from build123d import *

# Parameters (mm, degrees)
F0_W           = 200
F0_H           = 200
F1_DEPTH       = 20
F2_R           = 2.5
F3_W           = 180
F3_H           = 180
F4_DEPTH       = 2
F6_D           = 8
F6_CBORE_D     = 13
F6_CBORE_DEPTH = 8


with BuildPart() as f1:
    # F0 (on Top) → F1 (new body)
    with BuildSketch(Plane.XY):
        Rectangle(F0_W, F0_H)
    extrude(amount=F1_DEPTH)

    # F2
    f2_edges = [f1.edges().sort_by_distance(p)[0] for p in [
        (0, 100, 20),
        (100, 0, 20),
        (100, 100, 10),
        (0, 100, 0),
        (100, 0, 0),
        (-100, 0, 0),
        (-100, 0, 20),
        (-100, 100, 10),
        (100, -100, 10),
        (0, -100, 20),
        (0, -100, 0),
        (-100, -100, 10),
    ]]
    fillet(f2_edges, radius=F2_R)

    # F3 (on face) → F4 (cut)
    with BuildSketch(Plane.XY.offset(20)):
        Rectangle(F3_W, F3_H)
    extrude(amount=-F4_DEPTH, mode=Mode.SUBTRACT)

    # F6 (through all)
    with Locations(Plane.XY.offset(18)):
        with Locations((-50, 50), (50, 50), (50, -50), (-50, -50)):
            CounterBoreHole(F6_D / 2, F6_CBORE_D / 2, F6_CBORE_DEPTH)


solid = f1.part
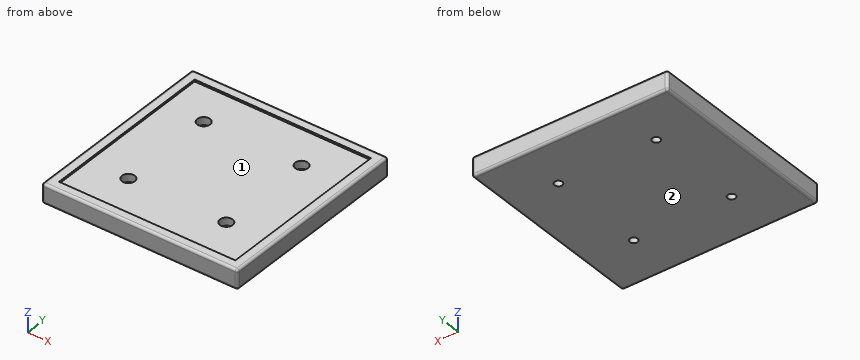
The listing builds one solid part. Answer for the finished solid, in the listing's coordinates (mm). Face numbers are marked on the shaded views. Give positions to 0.01 mm unless a question says otherwise; leave off trailing zeros. Write each loop counter-clockwise with the first axis right and the second up, starting at its lowest first coordinate (ties: lowest second). Pieces come first, ordered by that corner, then holes.
Item 1: Section A-A, the plane x = -50 is taken. Write down the section's boundary in (y, z), plus the area to 3 significant figures.
Item 2: Flat-ended cylindrical pins translate along their axes: P1, Ø10.5, axis at x = 50, y = -50, coming from the +Z side; P2, Ø21, axis at x = -50, y = -50, coming from the +Z side; P3, Ø1.6, axis at y = -37, z = 18.5, coming from the +X side. Find the tip coordinate at first contact, or state that the pin passes through.
Item 3: Determine the mould class of the marked faces 1 and 2 for opening direction Y: released by +Y, released by -Y, zero draft, split by the parting line, or undercut.
Item 4: Section C-C, the plane x = -83 is taken. Write down the section's boundary in (y, z).
Item 5: Find the intervals of material crossed by line 1 along Y through (x, z) = (-50, 13.25); line 2 along Y through (x, z) = (-50.5, 8.5); line 3 along Z through (x, y) = (-85, 41.5), in increasing order.
Completed:
1. outline: (-100, 2.5) arc R2.5 ccw to (-97.5, 0) - (-54, 0) - (-54, 10) - (-56.5, 10) - (-56.5, 18) - (-90, 18) - (-90, 20) - (-97.5, 20) arc R2.5 ccw to (-100, 17.5) - close; (-46, 0) - (46, 0) - (46, 10) - (43.5, 10) - (43.5, 18) - (-43.5, 18) - (-43.5, 10) - (-46, 10) - close; (54, 0) - (97.5, 0) arc R2.5 ccw to (100, 2.5) - (100, 17.5) arc R2.5 ccw to (97.5, 20) - (90, 20) - (90, 18) - (56.5, 18) - (56.5, 10) - (54, 10) - close
1. area: 3,270 mm2
2. P1: stops at z = 10
2. P2: stops at z = 18
2. P3: stops at x = 99.99
3. face 1: undercut
3. face 2: zero draft
4. outline: (-100, 2.5) arc R2.5 ccw to (-97.5, 0) - (97.5, 0) arc R2.5 ccw to (100, 2.5) - (100, 17.5) arc R2.5 ccw to (97.5, 20) - (90, 20) - (90, 18) - (-90, 18) - (-90, 20) - (-97.5, 20) arc R2.5 ccw to (-100, 17.5) - close
5. line 1: y = -100 to -56.5, -43.5 to 43.5, 56.5 to 100
5. line 2: y = -100 to -53.97, -46.03 to 46.03, 53.97 to 100
5. line 3: z = 0 to 18
